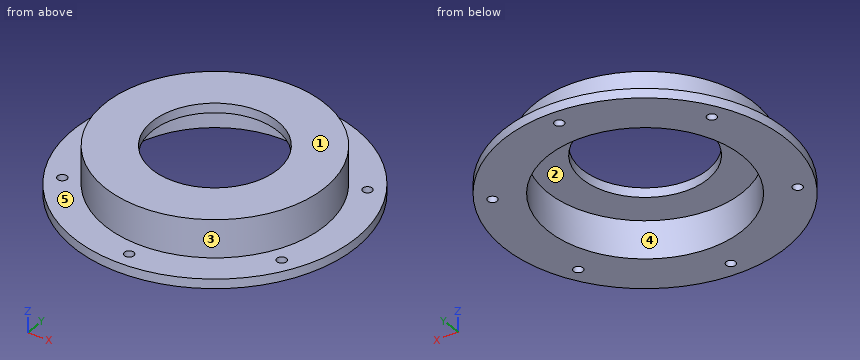
```python
from build123d import *

# Parameters (mm, degrees)
SKETCH1_R               = 45
BOSS_EXTRUDE3_DEPTH     = 3
SKETCH2_R               = 35
BOSS_EXTRUDE4_DEPTH     = 12
SKETCH3_R               = 31
CUT_EXTRUDE2_DEPTH      = 66.383484153
BOSS_EXTRUDE5_START     = -3
SKETCH4_R               = 35
SKETCH4_R_2             = 20
BOSS_EXTRUDE5_DEPTH     = 3
CUT_EXTRUDE3_DEPTH      = 65.761099435
CUT_EXTRUDE3_DEPTH_BACK = 65.761099435
SKETCH5_R               = 1.5


with BuildPart() as part:
    # Sketch1 → Boss-Extrude3 (new body)
    with BuildSketch(Plane.XY):
        Circle(SKETCH1_R)
    extrude(amount=BOSS_EXTRUDE3_DEPTH)

    # Sketch2 → Boss-Extrude4 (add)
    with BuildSketch(Plane.XY.offset(3)):
        Circle(SKETCH2_R)
    extrude(amount=BOSS_EXTRUDE4_DEPTH)

    # Sketch3 → Cut-Extrude2 (cut, through all)
    with BuildSketch(Plane.XY.offset(15)):
        Circle(SKETCH3_R)
    extrude(amount=-CUT_EXTRUDE2_DEPTH, mode=Mode.SUBTRACT)

    # Sketch4 → Boss-Extrude5 (add)
    with BuildSketch(Plane.XY.offset(15).offset(BOSS_EXTRUDE5_START)):
        Circle(SKETCH4_R)
        Circle(SKETCH4_R_2, mode=Mode.SUBTRACT)
    extrude(amount=BOSS_EXTRUDE5_DEPTH)

    # Sketch5 → Cut-Extrude3 (cut, two sides: drawn at the far end of the back side and taken through both)
    with BuildSketch(Plane.XY.offset(3).offset(-CUT_EXTRUDE3_DEPTH_BACK)):
        with Locations((0, 40)):
            Circle(SKETCH5_R)
        with Locations((34.641016151, 20)):
            Circle(SKETCH5_R)
        with Locations((34.641016151, -20)):
            Circle(SKETCH5_R)
        with Locations((0, -40)):
            Circle(SKETCH5_R)
        with Locations((-34.641016151, -20)):
            Circle(SKETCH5_R)
        with Locations((-34.641016151, 20)):
            Circle(SKETCH5_R)
    extrude(amount=CUT_EXTRUDE3_DEPTH + CUT_EXTRUDE3_DEPTH_BACK, mode=Mode.SUBTRACT)


solid = part.part
```
Input: part model. Units: mm. Frame: model coordinates. Face numbers are marked on the shaded views. A direction names the side the tool comes from. Give positions to 0.01 mm unless a question says otherwise; leave off trailing zeros. Order: outer loops, then holes, each group sorted by start corner. A loop starts at its lowest first (then second) coordinate and runs counter-clockwise, first axis right, second up. Notation, with made-up numbers: M -21.75,58.25 L 19.25,58.25 A11 cw 19.25,69.25 Z; hole C -2.75,-0.5 d8. An arc over 180 degrees is marked long. One line per question, with ' | ' between items. Start each with the question number.
1. Pull-direction query (X, two-part tool) for the marked faces 3, 4 and 5; classes: released by +X, released by -X, zero draft, split by the parting line, or undercut.
2. Section query C-C (z = 4.25). Return the cut outline in (x, y).
3. Access query for the marked faces 1 and 2. Directions: +Z, -Z, +X, -X, +Y, -Y. A direction counts if a zero-diameter tool reaches every point of the face in a straight line with its end or side. Return the directions, or none.
4. First-contact query: pin 1 Ø1 at (y, z) = (-22, 9.5) entering from -X; pin 2 Ø3 at (x, z) = (-6.5, 2) entering from +Y; pin 3 Ø3 at (y, z) = (33, 8) entering from +X. Flat tips, straight axial feed; report the tip coordinate or a pass-through.
5. Material intervals for probe 1 along Y at (x, z) = (-0.5, 10); probe 2 along X at (y, z) = (20, 1.1); probe 3 along Y at (x, z) = (0, 13.2), sorted ascending. Write a range as [from, to].
6. Section query D-D (y = -27.5). Return the cut outline in (x, z).
7. Section query B-B (y = 9.5). Return the cut outline in (x, z), and give its area (3 significant figures).
8. Section query A-A (x = 0). Return the cut outline in (y, z).
Here are the results:
1) face 3: split by the parting line | face 4: undercut | face 5: zero draft
2) outline: C 0,0 d70; hole C 0,0 d62
3) face 1: +Z, +X, -X, +Y, -Y | face 2: -Z
4) pin 1: x = -27.62 | pin 2: y = 44.72 | pin 3: x = 15.26
5) probe 1: [-35, -31], [31, 35] | probe 2: [-40.31, -36.14], [-33.14, -23.69], [23.69, 33.14], [36.14, 40.31] | probe 3: [-35, -20], [20, 35]
6) outline: M -35.62,0 L -14.31,0 L -14.31,12 L 14.31,12 L 14.31,0 L 35.62,0 L 35.62,3 L 21.65,3 L 21.65,15 L -21.65,15 L -21.65,3 L -35.62,3 Z
7) outline: M -43.99,0 L -29.51,0 L -29.51,12 L -17.6,12 L -17.6,15 L -33.69,15 L -33.69,3 L -43.99,3 Z; M 17.6,12 L 29.51,12 L 29.51,0 L 43.99,0 L 43.99,3 L 33.69,3 L 33.69,15 L 17.6,15 Z | area: 259 mm²
8) outline: M -45,0 L -41.5,0 L -41.5,3 L -45,3 Z; M -38.5,0 L -31,0 L -31,12 L -20,12 L -20,15 L -35,15 L -35,3 L -38.5,3 Z; M 20,12 L 31,12 L 31,0 L 38.5,0 L 38.5,3 L 35,3 L 35,15 L 20,15 Z; M 41.5,0 L 45,0 L 45,3 L 41.5,3 Z
